Here's how the part is built. I have some questions about the finished solid (model axes, mm). A direction names the side the tool comes from. Round coordinates to 2 decimals unless told otherwise and drop trailing zeros. Write each loop counter-clockwise with the first axis right and the second up, starting at its lowest first coordinate (ties: lowest second). Pieces come first, ordered by that corner, then holes. Notation, with made-up numbers: (11.25, -34.5) - (60.25, -34.5) arc R27 cw to (60.25, -5.5) - close; hole circle Ø9 at (39.5, -8). An arc over 180 degrees is marked (long way). One line per item, written item: value. Start each with the question number.
Item 1: For P1, Ø1, axis at y = -15.5, z = 70.5, coming from the -X side; P2, Ø8, axis at x = 50.5, z = 32.5, coming from the +Y side; P3, Ø8, axis at x = 77.5, y = 19.5, coming from the +Z side, each with a flat end and sliding along its axis, tell me the tip position at first contact or that it passes through.
Item 2: Imagine slicing it at A-A, the plane x = 0. Please give me the cut outline in (y, z), then the cut area to 3 significant figures.
Item 3: Imagine slicing it at B-B, the plane z = 37. Please give me the cut outline in (x, y), then the cut area to 3 significant figures.
Item 4: If I drill on line 1 (Y direction, x = 0, z = 34.5); line 2 (Y direction, x = 12.5, z = 30); line 3 (Z direction, x = -90, y = 9), over which ranges is the centre line in solid material (lowest first)?
Item 5: Thinking about a two-plate mould opening in Y: for faces 1 (the face through (-63.357, -5.326, 77.452)), 2 (the face through (-5.506, -24.796, 37.567)), 3 (the face through (-54, 0, 78.74)), which applies, released by +Y, released by -Y, zero draft, split by the parting line, or undercut?
Item 6: For faces 4 (the face through (63.357, -5.326, 77.452)), 5 (the face through (63.95, 5.18, 77.45)), 6 (the face through (-63.95, 5.18, 77.45)), 7 (the face through (54, 0, 78.74)), which set-ups out of +Z, -Z, +X, -X, +Y, -Y let a thin tool reach every point of the face, with its end or its side?
Item 7: Imagine slicing it at C-C, the plane z = 72. Please give me the cut outline in (x, y), then the cut area to 3 significant figures.
```python
from build123d import *

# Parameters (mm, degrees)
SKETCH1_R           = 101.6
SKETCH1_R_2         = 25.4
BOSS_EXTRUDE1_DEPTH = 76.2
FILLET1_R           = 7.62
BOSS_EXTRUDE2_DEPTH = 2.54


with BuildPart() as part:
    # Sketch1 → Boss-Extrude1 (new body)
    with BuildSketch(Plane.XY):
        Circle(SKETCH1_R)
        Circle(SKETCH1_R_2, mode=Mode.SUBTRACT)
    extrude(amount=BOSS_EXTRUDE1_DEPTH)

    # Fillet1
    fillet1_edges = [part.edges().sort_by_distance(p)[0] for p in [
        (-101.6, 0, 0),
        (-101.6, 0, 76.2),
    ]]
    fillet(fillet1_edges, radius=FILLET1_R)

    # Sketch2 → Boss-Extrude2 (add)
    with BuildSketch(Plane.XY.offset(76.2)):
        with BuildLine():
            add(Edge.make_bspline(
                [(42.436322164, 10.50404014), (34.587368685, 10.50404014), (34.587368685, 0)],
                knots=[0, 0, 0, 1.570796327, 1.570796327, 1.570796327], degree=2, weights=[1, 0.707106781, 1]))
            Line((34.587368685, 0), (84.872644329, 0))
            Line((84.872644329, 0), (42.436322164, 10.50404014))
        make_face()
        with BuildLine():
            Line((84.872644329, 0), (34.587368685, 0))
            add(Edge.make_bspline(
                [(34.587368685, 0), (34.587368685, -10.50404014), (42.436322164, -10.50404014)],
                knots=[1.570796327, 1.570796327, 1.570796327, 3.141592654, 3.141592654, 3.141592654], degree=2, weights=[1, 0.707106781, 1]))
            Line((42.436322164, -10.50404014), (84.872644329, 0))
        make_face()
    boss_extrude2 = extrude(amount=BOSS_EXTRUDE2_DEPTH)

    # Mirror1: Boss-Extrude2 across plane
    add(boss_extrude2.mirror(Plane(origin=(0, 0, 0), x_dir=(0, 0, 1), z_dir=(1, 0, 0))))


solid = part.part
```
Values follow:
1. P1: stops at x = -100.3
1. P2: stops at y = 90.33
1. P3: stops at z = 76.2
2. outline: (-101.6, 7.62) arc R7.62 ccw to (-93.98, 0) - (-25.4, 0) - (-25.4, 76.2) - (-93.98, 76.2) arc R7.62 ccw to (-101.6, 68.58) - close; (25.4, 0) - (93.98, 0) arc R7.62 ccw to (101.6, 7.62) - (101.6, 68.58) arc R7.62 ccw to (93.98, 76.2) - (25.4, 76.2) - close
2. area: 11,600 mm^2
3. outline: circle Ø203.2 at (0, 0); hole circle Ø50.8 at (0, 0)
3. area: 30,400 mm^2
4. line 1: y = -101.6 to -25.4, 25.4 to 101.6
4. line 2: y = -100.83 to -22.11, 22.11 to 100.83
4. line 3: z = 0 to 76.2
5. face 1: released by -Y
5. face 2: undercut
5. face 3: zero draft
6. face 4: +Z, +X, -Y
6. face 5: +Z, +X, +Y
6. face 6: +Z, -X, +Y
6. face 7: +Z, +X, -X, +Y, -Y
7. outline: circle Ø201.58 at (0, 0); hole circle Ø50.8 at (0, 0)
7. area: 29,900 mm^2
